```python
from build123d import *

# Parameters (mm, degrees)
BASE_FLANGE1_DEPTH = 1613
CUT_EXTRUDE1_REACH = 1620.23
FILLET1_R          = 3
CUT_EXTRUDE2_REACH = 1620.23
SKETCH7_R          = 4.5
LPATTERN1_COUNT    = 4
LPATTERN1_PITCH    = 529
CUT_EXTRUDE3_REACH = 1620.23
SKETCH8_R          = 3.25
CUT_EXTRUDE4_REACH = 1619.431
CUT_EXTRUDE5_REACH = 1619.431
SKETCH10_R         = 4.5
LPATTERN2_COUNT    = 3
LPATTERN2_PITCH    = 529
CUT_EXTRUDE6_REACH = 1619.431
SKETCH12_R         = 4.5


# Sheet-metal steps are written as plain solids
with BuildPart() as part:
    # Sketch1 → Base-Flange1 (new body)
    with BuildSketch(Plane(origin=(0, 0, 0), x_dir=(1, 0, 0), z_dir=(0, 1, 0))):
        with BuildLine():
            Line((-25, -120), (-25, -4.5))
            ThreePointArc((-25, -4.5), (-23.681980515, -1.318019485), (-20.5, 0))
            Line((-20.5, 0), (20.5, 0))
            ThreePointArc((20.5, 0), (23.681980515, -1.318019485), (25, -4.5))
            Line((25, -4.5), (25, -25))
            Line((25, -25), (22, -25))
            Line((22, -25), (22, -4.5))
            ThreePointArc((22, -4.5), (21.560660172, -3.439339828), (20.5, -3))
            Line((20.5, -3), (-20.5, -3))
            ThreePointArc((-20.5, -3), (-21.560660172, -3.439339828), (-22, -4.5))
            Line((-22, -4.5), (-22, -120))
            Line((-22, -120), (-25, -120))
        make_face()
    extrude(amount=BASE_FLANGE1_DEPTH)

    # Sketch6 → Cut-Extrude1 (cut, up to next)
    with BuildSketch(Plane.ZY.offset(25), mode=Mode.PRIVATE) as cut_extrude1_sk1:
        with BuildLine():
            Line((14.5, 16.25), (22.5, 16.25))
            ThreePointArc((22.5, 16.25), (25.75, 13), (22.5, 9.75))
            Line((22.5, 9.75), (14.5, 9.75))
            ThreePointArc((14.5, 9.75), (11.25, 13), (14.5, 16.25))
        make_face()
    cut_extrude1_tool1 = extrude(cut_extrude1_sk1.sketch, amount=-CUT_EXTRUDE1_REACH, mode=Mode.PRIVATE) & part.part
    cut_extrude1 = cut_extrude1_tool1.solids().sort_by_distance((-25, 13, 18.5))[0]
    add(cut_extrude1, mode=Mode.SUBTRACT)

    # Fillet1
    fillet1_edges = [part.edges().sort_by_distance(p)[0] for p in [
        (23.5, 0, 25),
        (-23.5, 0, 120),
        (23.5, 1613, 25),
        (-23.5, 1613, 120),
    ]]
    fillet(fillet1_edges, radius=FILLET1_R)

    # Sketch7 → Cut-Extrude2 (cut, up to next)
    with BuildSketch(Plane(origin=(25, 0, 0), x_dir=(0, 0, -1), z_dir=(1, 0, 0)), mode=Mode.PRIVATE) as cut_extrude2_sk1:
        with Locations((-15.5, 13)):
            Circle(SKETCH7_R)
    cut_extrude2_tool1 = extrude(cut_extrude2_sk1.sketch, amount=-CUT_EXTRUDE2_REACH, mode=Mode.PRIVATE) & part.part
    cut_extrude2 = cut_extrude2_tool1.solids().sort_by_distance((25, 13, 15.5))[0]
    add(cut_extrude2, mode=Mode.SUBTRACT)

    # LPattern1: Cut-Extrude1, Cut-Extrude2 ×4
    with Locations(*[(0, i * LPATTERN1_PITCH, 0) for i in range(1, LPATTERN1_COUNT)]):
        add(cut_extrude1, mode=Mode.SUBTRACT)
        add(cut_extrude2, mode=Mode.SUBTRACT)

    # Sketch8 → Cut-Extrude3 (cut, up to next)
    with BuildSketch(Plane.ZY.offset(25), mode=Mode.PRIVATE) as cut_extrude3_sk1:
        with Locations((107, 86.961524227)):
            Circle(SKETCH8_R)
    cut_extrude3_tool1 = extrude(cut_extrude3_sk1.sketch, amount=-CUT_EXTRUDE3_REACH, mode=Mode.PRIVATE) & part.part
    # Sketch8 → Cut-Extrude3 (cut, up to next)
    with BuildSketch(Plane.ZY.offset(25), mode=Mode.PRIVATE) as cut_extrude3_sk2:
        with Locations((77, 35)):
            Circle(SKETCH8_R)
    cut_extrude3_tool2 = extrude(cut_extrude3_sk2.sketch, amount=-CUT_EXTRUDE3_REACH, mode=Mode.PRIVATE) & part.part
    # Sketch8 → Cut-Extrude3 (cut, up to next)
    with BuildSketch(Plane.ZY.offset(25), mode=Mode.PRIVATE) as cut_extrude3_sk3:
        with Locations((107, 1230)):
            Circle(SKETCH8_R)
    cut_extrude3_tool3 = extrude(cut_extrude3_sk3.sketch, amount=-CUT_EXTRUDE3_REACH, mode=Mode.PRIVATE) & part.part
    # Sketch8 → Cut-Extrude3 (cut, up to next)
    with BuildSketch(Plane.ZY.offset(25), mode=Mode.PRIVATE) as cut_extrude3_sk4:
        with Locations((107, 1170)):
            Circle(SKETCH8_R)
    cut_extrude3_tool4 = extrude(cut_extrude3_sk4.sketch, amount=-CUT_EXTRUDE3_REACH, mode=Mode.PRIVATE) & part.part
    # Sketch8 → Cut-Extrude3 (cut, up to next)
    with BuildSketch(Plane.ZY.offset(25), mode=Mode.PRIVATE) as cut_extrude3_sk5:
        with Locations((107, 1530)):
            Circle(SKETCH8_R)
    cut_extrude3_tool5 = extrude(cut_extrude3_sk5.sketch, amount=-CUT_EXTRUDE3_REACH, mode=Mode.PRIVATE) & part.part
    # Sketch8 → Cut-Extrude3 (cut, up to next)
    with BuildSketch(Plane.ZY.offset(25), mode=Mode.PRIVATE) as cut_extrude3_sk6:
        with Locations((107, 1470)):
            Circle(SKETCH8_R)
    cut_extrude3_tool6 = extrude(cut_extrude3_sk6.sketch, amount=-CUT_EXTRUDE3_REACH, mode=Mode.PRIVATE) & part.part
    add(cut_extrude3_tool1.solids().sort_by_distance((-25, 86.961524, 107))[0], mode=Mode.SUBTRACT)
    add(cut_extrude3_tool2.solids().sort_by_distance((-25, 35, 77))[0], mode=Mode.SUBTRACT)
    add(cut_extrude3_tool3.solids().sort_by_distance((-25, 1230, 107))[0], mode=Mode.SUBTRACT)
    add(cut_extrude3_tool4.solids().sort_by_distance((-25, 1170, 107))[0], mode=Mode.SUBTRACT)
    add(cut_extrude3_tool5.solids().sort_by_distance((-25, 1530, 107))[0], mode=Mode.SUBTRACT)
    add(cut_extrude3_tool6.solids().sort_by_distance((-25, 1470, 107))[0], mode=Mode.SUBTRACT)

    # Sketch9 → Cut-Extrude4 (cut, up to next)
    with BuildSketch(Plane.XY.offset(3), mode=Mode.PRIVATE) as cut_extrude4_sk1:
        with BuildLine():
            Line((-16.5, 99.5), (-16.5, 124.5))
            ThreePointArc((-16.5, 124.5), (-1.5, 139.5), (13.5, 124.5))
            Line((13.5, 124.5), (13.5, 99.5))
            ThreePointArc((13.5, 99.5), (-1.5, 84.5), (-16.5, 99.5))
        make_face()
    cut_extrude4_tool1 = extrude(cut_extrude4_sk1.sketch, amount=-CUT_EXTRUDE4_REACH, mode=Mode.PRIVATE) & part.part
    # Sketch9 → Cut-Extrude4 (cut, up to next)
    with BuildSketch(Plane.XY.offset(3), mode=Mode.PRIVATE) as cut_extrude4_sk2:
        with BuildLine():
            Line((-16.5, 1187.5), (-16.5, 1212.5))
            ThreePointArc((-16.5, 1212.5), (-1.5, 1227.5), (13.5, 1212.5))
            Line((13.5, 1212.5), (13.5, 1187.5))
            ThreePointArc((13.5, 1187.5), (-1.5, 1172.5), (-16.5, 1187.5))
        make_face()
    cut_extrude4_tool2 = extrude(cut_extrude4_sk2.sketch, amount=-CUT_EXTRUDE4_REACH, mode=Mode.PRIVATE) & part.part
    # Sketch9 → Cut-Extrude4 (cut, up to next)
    with BuildSketch(Plane.XY.offset(3), mode=Mode.PRIVATE) as cut_extrude4_sk3:
        with BuildLine():
            Line((-16.5, 1487.5), (-16.5, 1512.5))
            ThreePointArc((-16.5, 1512.5), (-1.5, 1527.5), (13.5, 1512.5))
            Line((13.5, 1512.5), (13.5, 1487.5))
            ThreePointArc((13.5, 1487.5), (-1.5, 1472.5), (-16.5, 1487.5))
        make_face()
    cut_extrude4_tool3 = extrude(cut_extrude4_sk3.sketch, amount=-CUT_EXTRUDE4_REACH, mode=Mode.PRIVATE) & part.part
    add(cut_extrude4_tool1.solids().sort_by_distance((-1.5, 112, 3))[0], mode=Mode.SUBTRACT)
    add(cut_extrude4_tool2.solids().sort_by_distance((-1.5, 1200, 3))[0], mode=Mode.SUBTRACT)
    add(cut_extrude4_tool3.solids().sort_by_distance((-1.5, 1500, 3))[0], mode=Mode.SUBTRACT)

    # Sketch10 → Cut-Extrude5 (cut, up to next)
    with BuildSketch(Plane.XY.offset(3), mode=Mode.PRIVATE) as cut_extrude5_sk1:
        with Locations((0, 25)):
            Circle(SKETCH10_R)
    cut_extrude5_tool1 = extrude(cut_extrude5_sk1.sketch, amount=-CUT_EXTRUDE5_REACH, mode=Mode.PRIVATE) & part.part
    cut_extrude5 = cut_extrude5_tool1.solids().sort_by_distance((0, 25, 3))[0]
    add(cut_extrude5, mode=Mode.SUBTRACT)

    # LPattern2: Cut-Extrude5 ×3
    with Locations(*[(0, i * LPATTERN2_PITCH, 0) for i in range(1, LPATTERN2_COUNT)]):
        add(cut_extrude5, mode=Mode.SUBTRACT)

    # Sketch12 → Cut-Extrude6 (cut, up to next)
    with BuildSketch(Plane.XY.offset(3), mode=Mode.PRIVATE) as cut_extrude6_sk1:
        with Locations((0, 1588)):
            Circle(SKETCH12_R)
    cut_extrude6_tool1 = extrude(cut_extrude6_sk1.sketch, amount=-CUT_EXTRUDE6_REACH, mode=Mode.PRIVATE) & part.part
    add(cut_extrude6_tool1.solids().sort_by_distance((0, 1588, 3))[0], mode=Mode.SUBTRACT)


solid = part.part
```
Here's how the part is built. I have some questions about the finished solid (model axes, mm). A direction names the side the tool comes from. Coordinates: 2 decimals unless noted, no trailing zeros. Order: outer loops, then holes, each group sorted by start corner. A loop starts at its lowest first (then second) coordinate and runs counter-clockwise, first axis right, second up. Notation, with made-up numbers: (-38, -3.5) - (-20, -3.5) arc R31 cw to (-20, 33.5) - close; hole circle Ø6 at (-20, 17.25). An arc over 180 degrees is marked (long way). One line per question, with ' | ' between items. Start each with the question number.
1. Please list where these lines run through material, in increasing order: line 1 along Y through (x, z) = (-24.2, 107); line 2 along X through (y, z) = (901, 7.5); line 3 along Y through (x, z) = (-23.05, 77). Write a range as [from, to].
2. If we mould it in two halves opening along X, with no side actions, what happens to faces 3 (the flat face through (-25, 795, 63)), 4 (the flat face through (-24, 1613, 37)), 5 (the flat face through (0, 795, 3))? For each: released by +X, released by -X, zero draft, split by the parting line, or undercut.
3. I'm going to push flat-ended pins straight in: pin 1 Ø10.5 at (x, y) = (0, 1083) entering from +Z; pin 2 Ø7.5 at (y, z) = (1230, 107) entering from +X; pin 3 Ø3.5 at (y, z) = (1198.5, 1.5) entering from +X. Where does each tip first touch, or does it pass through?
4. If we section it at A-A (y = 979.5): Write out the boundary of the cut face in (x, z), and give its area (3 significant figures).
5. Which directions (+Z, -Z, +X, -X, +Y, -Y) give clear straight access to the entire face, cutting with the end or side of a thin tool? Please do faces 1 (the flat face through (-22, 795, 61)), 2 (the flat face through (-24, 0, 37)).
Model answer:
1) line 1: y = [0, 83.71], [90.21, 1166.75], [1173.25, 1226.75], [1233.25, 1466.75], [1473.25, 1526.75], [1533.25, 1613] | line 2: x = [-25, -22], [22, 25] | line 3: y = [0, 31.75], [38.25, 1613]
2) face 3: released by -X | face 4: zero draft | face 5: undercut
3) pin 1: stops at z = 3 | pin 2: stops at x = -22 | pin 3: stops at x = 24.82
4) outline: (-25, 4.5) arc R4.5 ccw to (-20.5, 0) - (20.5, 0) arc R4.5 ccw to (25, 4.5) - (25, 25) - (22, 25) - (22, 4.5) arc R1.5 cw to (20.5, 3) - (-20.5, 3) arc R1.5 cw to (-22, 4.5) - (-22, 120) - (-25, 120) - close | area: 559 mm²
5) face 1: +Z, +Y, -Y | face 2: +Z, -Z, +X, -X, -Y
